Build history of the part. All positions in model axes, mm. A direction names the side the tool comes from. Round coordinates to 2 decimals unless told otherwise and drop trailing zeros. Loops run counter-clockwise (first coordinate to the right, second up) from the corner with the lowest first, then second, coordinate; pieces in that order, holes last.
from build123d import *

# Parameters (mm, degrees)
BOX012_W               = 4
BOX012_H               = 10
BOX012_DEPTH           = 1.4
CYLINDER012_R          = 0.7
CYLINDER012_DEPTH      = 10
CYLINDER012_ROLL_ANGLE = 90
CYLINDER013_R          = 0.7
CYLINDER013_DEPTH      = 10
CYLINDER013_ROLL_ANGLE = 90
BOX011_W               = 21
BOX011_H               = 4
BOX011_DEPTH           = 10
CHAMFER003_SIZE        = 3.8
CYLINDER014_R          = 1
CYLINDER014_DEPTH      = 5
CYLINDER014_ROLL_ANGLE = 90
BOX010_W               = 15.5
BOX010_H               = 2.7
BOX010_DEPTH           = 5
CHAMFER001_SIZE        = 1.5
CHAMFER002_SIZE        = 1.2
CHAMFER004_SIZE        = 0.9


with BuildPart() as cube007:
    # Box012 → Box012 (new body)
    with BuildSketch(Plane(origin=(-7, -24.5, -39.3), x_dir=(1, 0, 0), z_dir=(0, 0, 1))):
        with Locations((2, 5)):
            Rectangle(BOX012_W, BOX012_H)
    extrude(amount=BOX012_DEPTH)


with BuildPart() as cylinder003:
    # Cylinder012 → Cylinder012 (new body)
    with BuildSketch(Plane.XY):
        Circle(CYLINDER012_R)
    extrude(amount=CYLINDER012_DEPTH)


with BuildPart() as cylinder003_1:
    # Cylinder012 roll: moved
    add(cylinder003.part.rotate(Axis((0, 0, 0), (1, 0, 0)), CYLINDER012_ROLL_ANGLE))


with BuildPart() as cylinder003_2:
    # Cylinder012 placement: moved
    add(cylinder003_1.part.moved(Location((-3, -14.5, -38.6))))


with BuildPart() as cylinder004:
    # Cylinder013 → Cylinder013 (new body)
    with BuildSketch(Plane.XY):
        Circle(CYLINDER013_R)
    extrude(amount=CYLINDER013_DEPTH)


with BuildPart() as cylinder004_1:
    # Cylinder013 roll: moved
    add(cylinder004.part.rotate(Axis((0, 0, 0), (1, 0, 0)), CYLINDER013_ROLL_ANGLE))


with BuildPart() as cylinder004_2:
    # Cylinder013 placement: moved
    add(cylinder004_1.part.moved(Location((-7, -14.5, -38.6))))


with BuildPart() as fusion007005:
    # Fusion007005 base: copy of Cylinder004
    add(cylinder004_2.part)

    # Fusion007005: union Cube007, Cylinder003
    add(cube007.part)
    add(cylinder003_2.part)


with BuildPart() as fusion007005_1:
    # Fusion007005 placement: moved
    add(fusion007005.part.moved(Location((7, 0, 0))))


with BuildPart() as fusion007006:
    # Fusion007006 base: copy of Cylinder004
    add(cylinder004_2.part)

    # Fusion007006: union Cube007, Cylinder003
    add(cube007.part)
    add(cylinder003_2.part)


with BuildPart() as chamfer003:
    # Box011 → Box011 (new body)
    with BuildSketch(Plane(origin=(-15, -21, -44), x_dir=(1, 0, 0), z_dir=(0, 0, 1))):
        with Locations((10.5, 2)):
            Rectangle(BOX011_W, BOX011_H)
    extrude(amount=BOX011_DEPTH)

    # Cut007: cut Fusion007006
    add(fusion007006.part, mode=Mode.SUBTRACT)

    # Cut008: cut Fusion007005
    add(fusion007005_1.part, mode=Mode.SUBTRACT)

    # Chamfer003
    chamfer003_edges = [chamfer003.edges().sort_by_distance(p)[0] for p in [
        (-15, -21, -39),
    ]]
    chamfer(chamfer003_edges, length=CHAMFER003_SIZE)


with BuildPart() as cylinder005:
    # Cylinder014 → Cylinder014 (new body)
    with BuildSketch(Plane.XY):
        Circle(CYLINDER014_R)
    extrude(amount=CYLINDER014_DEPTH)


with BuildPart() as cylinder005_1:
    # Cylinder014 roll: moved
    add(cylinder005.part.rotate(Axis((0, 0, 0), (1, 0, 0)), CYLINDER014_ROLL_ANGLE))


with BuildPart() as cylinder005_2:
    # Cylinder014 placement: moved
    add(cylinder005_1.part.moved(Location((-21.5, -13.5, -38.75))))


with BuildPart() as chamfer004:
    # Box010 → Box010 (new body)
    with BuildSketch(Plane(origin=(-24, -17.5, -41.25), x_dir=(1, 0, 0), z_dir=(0, 0, 1))):
        with Locations((7.75, 1.35)):
            Rectangle(BOX010_W, BOX010_H)
    extrude(amount=BOX010_DEPTH)

    # Cut009: cut Cylinder005
    add(cylinder005_2.part, mode=Mode.SUBTRACT)

    # Chamfer001
    chamfer001_edges = [chamfer004.edges().sort_by_distance(p)[0] for p in [
        (-24, -16.15, -36.25),
        (-24, -16.15, -41.25),
    ]]
    chamfer(chamfer001_edges, length=CHAMFER001_SIZE)

    # Chamfer002
    chamfer002_edges = [chamfer004.edges().sort_by_distance(p)[0] for p in [
        (-15.5, -17.5, -41.25),
        (-15.5, -17.5, -36.25),
    ]]
    chamfer(chamfer002_edges, length=CHAMFER002_SIZE)

    # Fusion007007: union Chamfer003
    add(chamfer003.part)

    # Chamfer004
    chamfer004_edges = [chamfer004.edges().sort_by_distance(p)[0] for p in [
        (-11.75, -17, -36.95),
        (-8.5, -16.65, -40.9),
    ]]
    chamfer(chamfer004_edges, length=CHAMFER004_SIZE)


solid = chamfer004.part
(1) Slice it at C-C on z = -38.75. List the corners of the cut face in (x, y).
Responses:
outline: (-24, -17.5) - (-22.5, -17.5) - (-22.5, -14.8) - (-24, -14.8) - close; (-20.5, -17.5) - (-14.7, -17.5) - (-11.2, -21) - (-7.68, -21) - (-7.68, -17) - (-8.5, -17) - (-8.5, -14.8) - (-20.5, -14.8) - close; (-2.32, -21) - (-0.68, -21) - (-0.68, -17) - (-2.32, -17) - close; (4.68, -21) - (6, -21) - (6, -17) - (4.68, -17) - close
(2) Pull direction X, two halves, no side cores. Call faces 1 (the face through (2, -19, -37.9)), 2 (the face through (-3, -21, -40)), 3 (the face through (-23.24, -15.87, -40.51)): +X half, -X half, draft (parallel to the pull), parting line (faces both ways), or undercut.
Responses:
face 1: undercut
face 2: draft
face 3: -X half
(3) Probe line 1 (X direction, y = -16.9, z = -38.75); line 2 (Z direction, x = -21.5, y = -16); line 3 (Z direction, x = -6.25, y = -20.5). List the from-to ranges inside material, lowest first.
Responses:
line 1: x = -24 to -22.5, -20.5 to -8.5
line 2: z = -41.25 to -39.75, -37.75 to -36.25
line 3: z = -44 to -39.3, -37.9 to -34
(4) Which spindle directions (+Z, -Z, +X, -X, +Y, -Y) get a long thin tool onto all of the face, cutting with end or side? Do faces 4 (the face through (-16, -16, -41.25)), 5 (the face through (-16, -16, -36.25)), 6 (the face through (-19, -17.5, -39)), 7 (the face through (-5, -19, -37.9)). Say none if no direction does.
Responses:
face 4: -Z, +X, -X, +Y
face 5: +Z, +X, -X, +Y
face 6: +Z, -Z, -X, -Y
face 7: +Y, -Y
(5) Slice it at A-A on x = 3.5. List the corners of the cut face in (y, z), plus the area to 3 significant figures.
Responses:
outline: (-21, -44) - (-17, -44) - (-17, -39.3) - (-21, -39.3) - close; (-21, -37.9) - (-17, -37.9) - (-17, -34) - (-21, -34) - close
area: 34.4 mm2
(6) Slice it at D-D on x = -21.5. List the corners of the cut face in (y, z).
Responses:
outline: (-17.5, -40.05) - (-16.3, -41.25) - (-14.8, -41.25) - (-14.8, -39.75) - (-17.5, -39.75) - close; (-17.5, -37.75) - (-14.8, -37.75) - (-14.8, -36.25) - (-16.3, -36.25) - (-17.5, -37.45) - close
(7) Slice it at B-B on y = -19. List the corners of the cut face in (x, z), plus the area to 3 significant figures.
Responses:
outline: (-13.2, -44) - (6, -44) - (6, -34) - (-13.2, -34) - close; hole (-7, -39.3) - (-3, -39.3) arc R0.7 ccw to (-3, -37.9) - (-7, -37.9) arc R0.7 ccw to start; hole (0, -39.3) - (4, -39.3) arc R0.7 ccw to (4, -37.9) - (0, -37.9) arc R0.7 ccw to start
area: 178 mm2
(8) Pin check, flat tips, straight feed: P1, Ø3, axis at x = -14.5, z = -43, coming from the +Y side; P2, Ø1.7, axis at x = -17.5, y = -15.5, coming from the +Z side; P3, Ø3, axis at x = -18, z = -38.5, coming from the -Y side. Stop position of each tip, or through.
Responses:
P1: stops at y = -17
P2: stops at z = -36.25
P3: stops at y = -17.5
